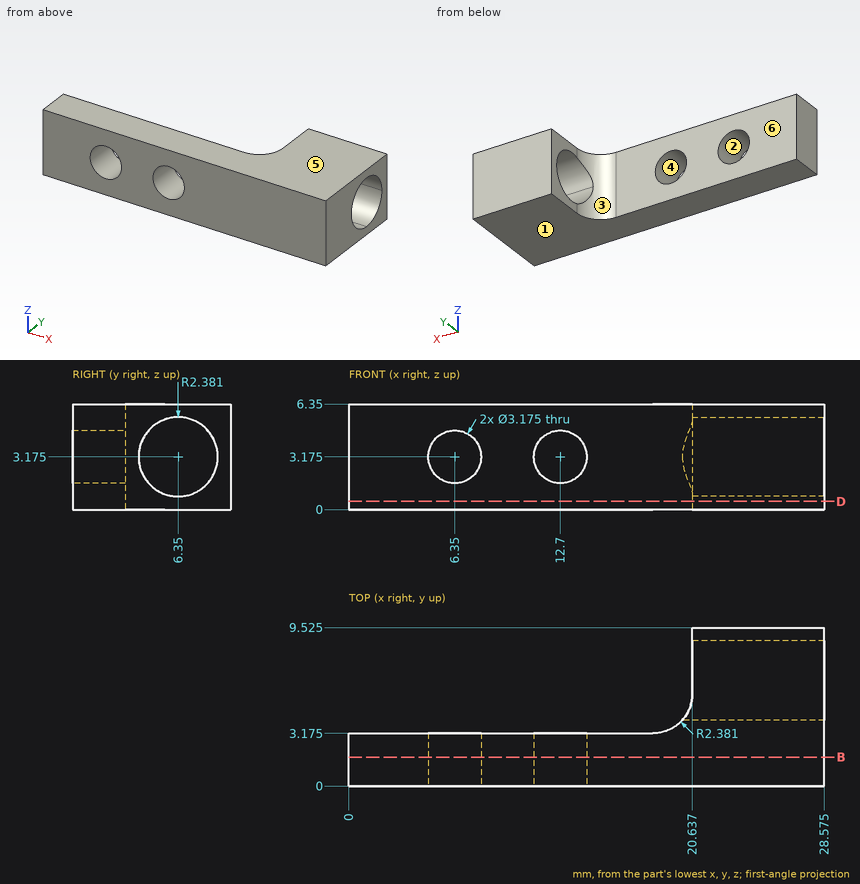
Geometry: see drawing. Coordinates: mm, zero at the bounding-box minimum. A direction names the side the tool comes from. Give positions to 0.01 mm unless a question says otherwise; leave off trailing zeros. Loops run counter-clockwise (first coordinate to the right, second up) from the corner with the lowest first, then second, coordinate; pieces in that order, holes last. Notation, with made-up numbers: (89.25, 49) -> (129.25, 49) arc R21 cw to (129.25, 69) -> close; hole circle Ø3 at (16.25, -26.5). An arc over 180 degrees is marked (long way). Answer as a JSON object with one key per item and string values. Group by question number.
Item 1: Cut plane B-B, the plane y = 1.75. State how many separate pieces and enclosed holes the cut face has, and give its area (3 significant figures).
Item 2: Line query: probe 1 along X at (y, z) = (1, 3.75) (1 decimal); probe 2 along Y at (x, z) = (3.75, 4) (1 decimal); probe 3 along Y at (x, z) = (27, 3) (1 decimal). Output: solid intervals per line, ascending.
Item 3: Cut plane D-D, the plane z = 0.5. Return the cut outline in (x, y) (1 decimal).
Item 4: Pin query (flat end, axial travel): P1, Ø1, axis at y = 4, z = 2, coming from the -X side (1 decimal); P2, Ø3, axis at y = 7.5, z = 2, coming from the -X side. Return the tip coordinate at first contact, or that it passes through.
Item 5: Pull-direction query (X, two-part tool) for the marked faces 1, 2, 3 and 4; classes: released by +X, released by -X, zero draft, split by the parting line, or undercut.
Item 6: Reachability of the marked faces 5 and 6 from +Z, -Z, +X, -X, +Y, -Y: full face, straight path, thin tool, end or side. Return the list, or none.
Checks:
{
 "1": {"separate pieces": "1", "enclosed holes": "2", "area": "166 mm²"},
 "2": {"probe 1": "x = 0 to 4.9, 7.8 to 11.2, 14.2 to 28.6", "probe 2": "y = 0 to 3.2", "probe 3": "y = 0 to 4, 8.7 to 9.5"},
 "3": {"outline": "(0, 0) -> (28.6, 0) -> (28.6, 9.5) -> (20.6, 9.5) -> (20.6, 5.6) arc R2.4 cw to (18.3, 3.2) -> (0, 3.2) -> close"},
 "4": {"P1": "stops at x = 19.5", "P2": "stops at x = 20.64"},
 "5": {"face 1": "zero draft", "face 2": "undercut", "face 3": "released by -X", "face 4": "undercut"},
 "6": {"face 5": "+Z, +X, -X, +Y, -Y", "face 6": "+Z, -Z, -X, +Y"}
}
